Here's the drawing with two shaded views (mm, measured from the low corner). I have some questions. A direction names the side the tool comes from. Coordinates: 2 decimals unless noted, no trailing zeros. Order: outer loops, then holes, each group sorted by start corner. A loop starts at its lowest first (then second) coordinate and runs counter-clockwise, first axis right, second up. Notation, with made-up numbers: (-37.5, -38) -> (0.5, -38) arc R13 cw to (0.5, -29) -> close; hole circle Ø1 at (-4, 43.25). An arc over 180 degrees is marked (long way). Answer in a Markdown table with one row per item. Add a question column.
1. Imagine slicing it at C-C on z = 12.75. Write out the boundary of the cut face in (x, y).
2. Will this pin go through, and if not, where does the flat tip stop? pin 1 (6 mm diameter, centred on x = 32.5, z = 10, fed in from +Y).
3. If I drill on line 1 along Y through (x, z) = (51, 8.5); line 2 along X through (y, z) = (16.5, 7.25); line 3 along X through (y, z) = (14.5, 22.75), over which ranges is the centre line in solid material (lowest first)? Write a range as [from, to].
4. We'd pull the mould along Y, two halves only. Please class the marked faces 1, 2 and 3: pulls with the +Y half, pulls with the -Y half, needs draft (parallel to the pull), parting line crosses it, or undercut.
5. On a 3-axis mill with a long thin cutter (end or side, diameter ignored), from which of +Z, -Z, +X, -X, +Y, -Y can I reach the whole of each face in a straight line? I mean the marked faces 4 and 5. Say none if no direction works.
6. Imagine slicing it at A-A on y = 13. Write out the boundary of the cut face in (x, z).
7. Imagine slicing it at B-B on x = 13. Write out the boundary of the cut face in (y, z).
8. Imagine slicing it at D-D on y = 10. Write out the boundary of the cut face in (x, z), plus the area to 3 significant figures.
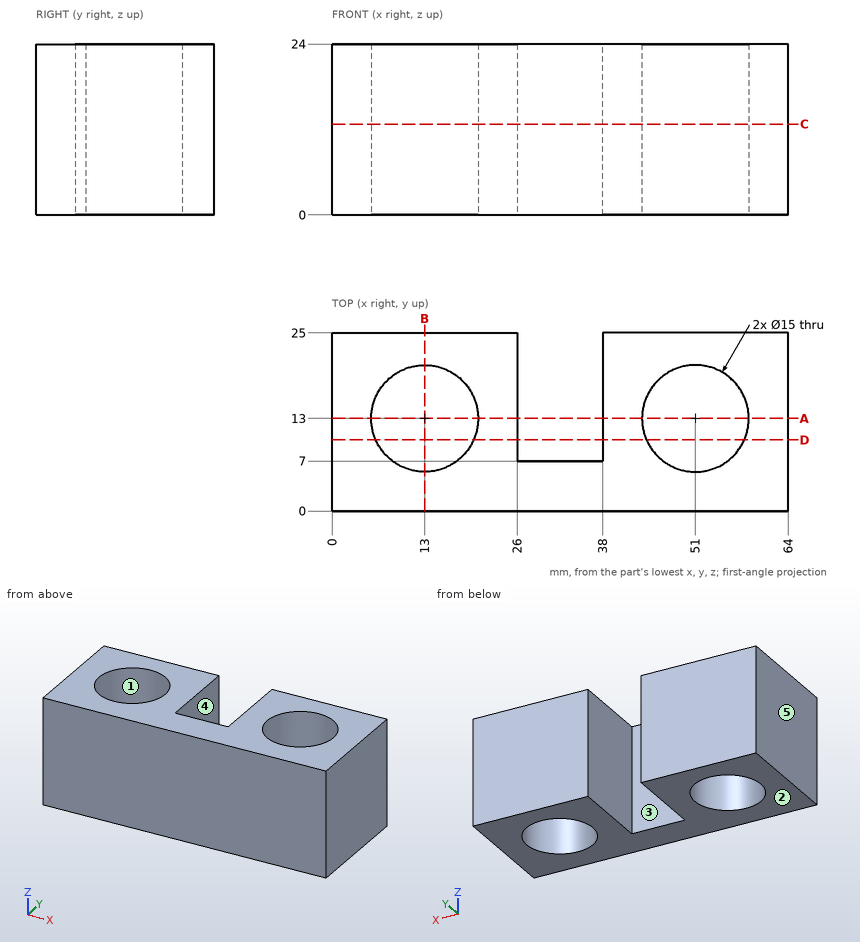
Answers follow:
| question | item | result |
|---|---|---|
| 1 | outline | (0, 0) -> (64, 0) -> (64, 25) -> (38, 25) -> (38, 7) -> (26, 7) -> (26, 25) -> (0, 25) -> close; hole circle Ø15 at (13, 13); hole circle Ø15 at (51, 13) |
| 2 | pin 1 | stops at y = 7 |
| 3 | line 1 | y = [0, 5.5], [20.5, 25] |
| 3 | line 2 | x = [0, 6.37], [19.63, 26], [38, 44.37], [57.63, 64] |
| 3 | line 3 | x = [0, 5.65], [20.35, 26], [38, 43.65], [58.35, 64] |
| 4 | face 1 | undercut |
| 4 | face 2 | needs draft |
| 4 | face 3 | pulls with the +Y half |
| 5 | face 4 | +Z, -Z, +Y |
| 5 | face 5 | +Z, -Z, -X, +Y, -Y |
| 6 | outline | (0, 0) -> (5.5, 0) -> (5.5, 24) -> (0, 24) -> close; (20.5, 0) -> (26, 0) -> (26, 24) -> (20.5, 24) -> close; (38, 0) -> (43.5, 0) -> (43.5, 24) -> (38, 24) -> close; (58.5, 0) -> (64, 0) -> (64, 24) -> (58.5, 24) -> close |
| 7 | outline | (0, 0) -> (5.5, 0) -> (5.5, 24) -> (0, 24) -> close; (20.5, 0) -> (25, 0) -> (25, 24) -> (20.5, 24) -> close |
| 8 | outline | (0, 0) -> (6.13, 0) -> (6.13, 24) -> (0, 24) -> close; (19.87, 0) -> (26, 0) -> (26, 24) -> (19.87, 24) -> close; (38, 0) -> (44.13, 0) -> (44.13, 24) -> (38, 24) -> close; (57.87, 0) -> (64, 0) -> (64, 24) -> (57.87, 24) -> close |
| 8 | area | 588 mm² |
